from build123d import *

# Parameters (mm, degrees)
F1_DEPTH = 6.35


with BuildPart() as f1:
    # F0 (on Right) → F1 (new body)
    with BuildSketch(Plane.YZ):
        Polygon((63.5, 25.4), (57.15, 25.4), (50.8, 25.4), (44.45, 25.4), (38.1, 25.4), (31.75, 25.4), (25.4, 25.4), (19.05, 25.4), (19.05, 19.05), (12.7, 19.05), (6.35, 19.05), (0, 19.05), (-6.35, 19.05), (-12.7, 19.05), (-19.05, 19.05), (-19.05, 25.4), (-25.4, 25.4), (-31.75, 25.4), (-38.1, 25.4), (-44.45, 25.4), (-50.8, 25.4), (-63.5, 25.4), (-63.5, 12.7), (-57.15, 12.7), (-57.15, 6.35), (-57.15, 0), (-57.15, -6.35), (-57.15, -12.7), (-63.5, -12.7), (-63.5, -19.05), (-63.5, -25.4), (-50.8, -25.4), (-44.45, -25.4), (-44.45, 6.35), (44.45, 6.35), (44.45, -25.4), (50.8, -25.4), (63.5, -25.4), (63.5, -19.05), (63.5, -12.7), (57.15, -12.7), (57.15, -6.35), (57.15, 0), (57.15, 6.35), (57.15, 12.7), (63.5, 12.7), align=None)
    extrude(amount=-F1_DEPTH)


solid = f1.part
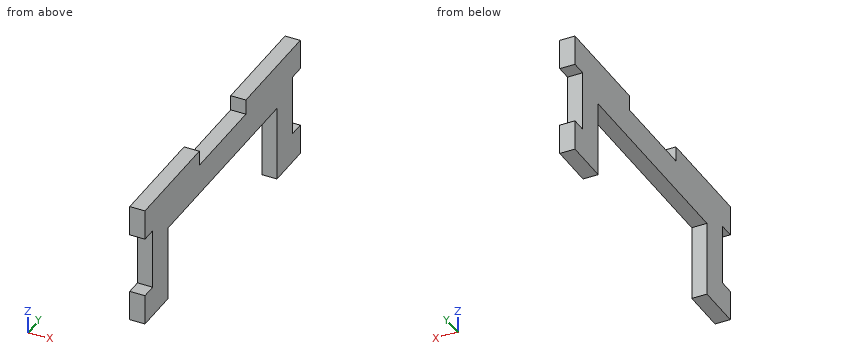
The listing builds one solid part. Answer for the finished solid, in the listing's coordinates (mm). Coordinates: 2 decimals unless noted, no trailing zeros. Loops run counter-clockwise (first coordinate to the right, second up) from the corner with the lowest first, then second, coordinate; pieces in that order, holes last. Notation, with made-up numbers: (23.25, 76) -> (80.25, 76) arc R14 cw to (80.25, 101) -> close; hole circle Ø1 at (-6, 52). An arc over 180 degrees is marked (long way). Answer in a Markdown table with one row per item. Add a question column.
1. The part is cut by section A-A, the plane z = -5. Write down the section's boundary in (x, y), then the cut area to 3 significant figures.
2. Flat-ended cylindrical pins translate along their axes: P1, Ø1.9, axis at x = -3, y = -0.5, coming from the -Z side; P2, Ø2, axis at x = -5.5, z = -1, coming from the +Y side; P3, Ø3, axis at x = -3.5, z = -5, coming from the -Y side. Find the tip coordinate at first contact, or state that the pin passes through.
3. The part is cut by section D-D, the plane z = -14. Write down the section's boundary in (x, y), then the cut area to 3 significant figures.
4. The part is cut by section B-B, the plane x = -4.5. Write down the section's boundary in (y, z).
5. Consider line 1 (Y direction, x = -3, z = -15); line 2 (Y direction, x = -5.75, z = -4.5); line 3 (Z direction, x = -3, y = 9.5). Determine where each line is inside the solid, lowest interval first. Write a range as [from, to].
6. The part is cut by section C-C, the plane y = 7.5. Write down the section's boundary in (x, z).
Answer below:
| question | item | result |
|---|---|---|
| 1 | outline | (-6.35, -57.15) -> (0, -57.15) -> (0, -44.45) -> (-6.35, -44.45) -> close; (-6.35, 44.45) -> (0, 44.45) -> (0, 57.15) -> (-6.35, 57.15) -> close |
| 1 | area | 161 mm2 |
| 2 | P1 | z = 6.35 |
| 2 | P2 | y = 57.15 |
| 2 | P3 | y = -57.15 |
| 3 | outline | (-6.35, -63.5) -> (0, -63.5) -> (0, -44.45) -> (-6.35, -44.45) -> close; (-6.35, 44.45) -> (0, 44.45) -> (0, 63.5) -> (-6.35, 63.5) -> close |
| 3 | area | 242 mm2 |
| 4 | outline | (-63.5, -25.4) -> (-44.45, -25.4) -> (-44.45, 6.35) -> (44.45, 6.35) -> (44.45, -25.4) -> (63.5, -25.4) -> (63.5, -12.7) -> (57.15, -12.7) -> (57.15, 12.7) -> (63.5, 12.7) -> (63.5, 25.4) -> (19.05, 25.4) -> (19.05, 19.05) -> (-19.05, 19.05) -> (-19.05, 25.4) -> (-63.5, 25.4) -> (-63.5, 12.7) -> (-57.15, 12.7) -> (-57.15, -12.7) -> (-63.5, -12.7) -> close |
| 5 | line 1 | [-63.5, -44.45], [44.45, 63.5] |
| 5 | line 2 | [-57.15, -44.45], [44.45, 57.15] |
| 5 | line 3 | [6.35, 19.05] |
| 6 | outline | (-6.35, 6.35) -> (0, 6.35) -> (0, 19.05) -> (-6.35, 19.05) -> close |
